CAD build for the part. Positions are in the model's coordinates, mm. Give positions to 0.01 mm unless a question says otherwise; leave off trailing zeros. Write each loop counter-clockwise with the first axis right and the second up, starting at its lowest first coordinate (ties: lowest second). Pieces come first, ordered by that corner, then holes. Notation, with made-up numbers: (-15.75, 83) - (13.25, 83) arc R26 ccw to (13.25, 116) - close; hole circle Ø5 at (48, 85.5). An arc over 180 degrees is marked (long way). Answer as a JSON object with one key per item and string values.
from build123d import *

# Parameters (mm, degrees)
BOSS_EXTRUDE2_DEPTH = 15
FILLET4_START       = -11
FILLET4_DEPTH       = 22
SKETCH2_R           = 1.75
CUT_EXTRUDE1_DEPTH  = 32
SKETCH3_R           = 3
CUT_EXTRUDE2_DEPTH  = 47


with BuildPart() as part:
    # Sketch1 → Boss-Extrude2 (new body)
    with BuildSketch(Plane.XY):
        with BuildLine():
            Line((157.5, -10), (157.5, 10))
            Line((157.5, 10), (0, 15))
            ThreePointArc((0, 15), (-15, 0), (0, -15))
            Line((0, -15), (157.5, -10))
        make_face()
    extrude(amount=BOSS_EXTRUDE2_DEPTH)

    # Fillet4: read off the stored shape, not the designer's step
    # Fillet4 outline → Fillet4 (cut)
    with BuildSketch(Plane(origin=(0, 0, 0), x_dir=(1, 0, 0), z_dir=(0, 1, 0)).offset(FILLET4_START)):
        with BuildLine():
            ThreePointArc((150, 0), (155.303300859, -2.196699141), (157.5, -7.5))
            Line((157.5, -7.5), (157.5, 0))
            Line((157.5, 0), (150, 0))
        make_face()
        with BuildLine():
            ThreePointArc((157.5, -7.5), (155.303300859, -12.803300859), (150, -15))
            Line((150, -15), (157.5, -15))
            Line((157.5, -15), (157.5, -7.5))
        make_face()
    extrude(amount=FILLET4_DEPTH, mode=Mode.SUBTRACT)

    # Sketch2 → Cut-Extrude1 (cut)
    with BuildSketch(Plane.XY.offset(15)):
        with Locations((142.197100849, 0)):
            Circle(SKETCH2_R)
    extrude(amount=-CUT_EXTRUDE1_DEPTH, mode=Mode.SUBTRACT)

    # Sketch3 → Cut-Extrude2 (cut)
    with BuildSketch(Plane.XY.offset(15)):
        Circle(SKETCH3_R)
    extrude(amount=-CUT_EXTRUDE2_DEPTH, mode=Mode.SUBTRACT)


solid = part.part
Item 1: Cut at C-C (x = 126). Give the cut face in (y, z), and give its area (3 significant figures).
Entries:
{"outline": "(-11, 0) - (11, 0) - (11, 15) - (-11, 15) - close", "area": "330 mm2"}
Item 2: Cut at A-A (y = 0). Give the cut face in (x, z), and give its area (3 significant figures).
Entries:
{"outline": "(-15, 0) - (-3, 0) - (-3, 15) - (-15, 15) - close; (3, 0) - (140.45, 0) - (140.45, 15) - (3, 15) - close; (143.95, 0) - (150, 0) arc R7.5 ccw to (150, 15) - (143.95, 15) - close", "area": "2,420 mm2"}
Item 3: Cut at D-D (y = 7.5). Give the cut face in (x, z), and give its area (3 significant figures).
Entries:
{"outline": "(-12.99, 0) - (150, 0) arc R7.5 ccw to (150, 15) - (-12.99, 15) - close", "area": "2,530 mm2"}
Item 4: Cut at B-B (z = 3.75). Give the cut face in (x, y).
Entries:
{"outline": "(0, -15) - (156.5, -10.03) - (156.5, 10.03) - (0, 15) arc R15 ccw to start; hole circle Ø6 at (0, 0); hole circle Ø3.5 at (142.2, 0)"}
Item 5: Probe line 1 (Y direction, x = 0, z = 9.5); line 2 (X direction, y = 2, z = 11.5); line 3 (Y direction, x = 14, z = 6). List the from-to ranges inside material, lowest first. Write a range as from..to.
Entries:
{"line 1": "-15..-3, 3..15", "line 2": "-14.87..-2.24, 2.24..156.34", "line 3": "-14.56..14.56"}
Item 6: Flat gauge pins, fed straight in: P1, Ø2, axis at x = 142.2, y = 0, coming from the +Z side; P2, Ø3, axis at x = 122, z = 2.5, coming from the -Y side; P3, Ø8, axis at y = 4.5, z = 2, coming from the -X side; P4, Ø4, axis at y = 5.5, z = 11, coming from the +X side. Where does each tip first touch, or does it go through?
Entries:
{"P1": "through", "P2": "y = -11.17", "P3": "x = -14.99", "P4": "x = 157.35"}
Item 7: Mould opens along Y. For faces 1 (the cylindrical face through (-3, 0, 8)), 2 (the cylindrical face through (-15, 0, 7)), 3 (the flat face through (66, 0, 0)) say: +Y half, -Y half, draft (parallel to the pull), parting line (faces both ways), or undercut.
Entries:
{"face 1": "undercut", "face 2": "parting line", "face 3": "draft"}
